Study the drawing (mm; zero at the part's minimum x, y, z) and answer. A direction names the side the tool comes from. Coordinates: 2 decimals unless noted, no trailing zeros. Order: outer loops, then holes, each group sorted by start corner. A loop starts at its lowest first (then second) coordinate and runs counter-clockwise, first axis right, second up. Notation, with made-up numbers: (88, 5.25) -> (101, 5.25) arc R17 ccw to (101, 36.25) -> close; hole circle Ø1 at (45, 71.5). An arc over 180 degrees is marked (long way). One line per question, with ' | ' between items.
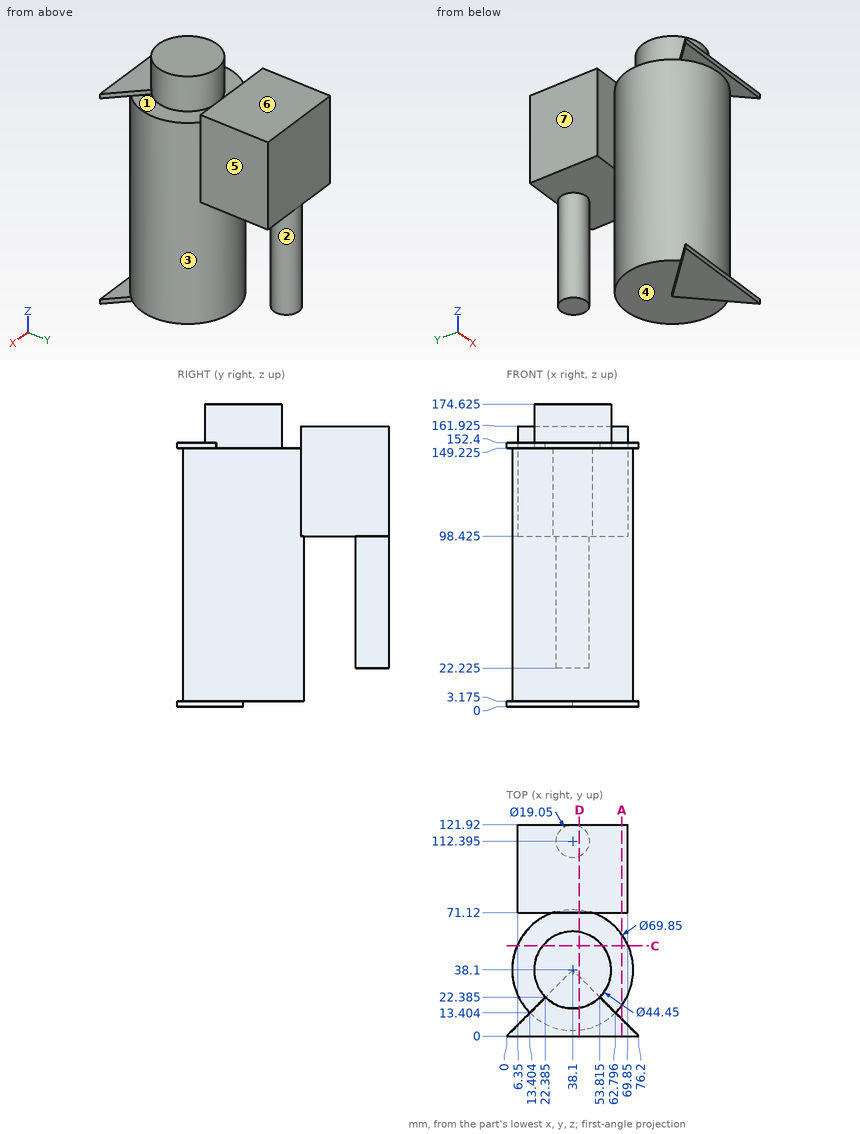
Item 1: Each of these flat-tipped pins is pushed along its axis until it touches: pin 1 Ø1.5 at (y, z) = (30, 156.5) entering from +X (1 decimal); pin 2 Ø10.5 at (x, y) = (52.5, 4.5) entering from -Z; pin 3 Ø1.5 at (y, z) = (55, 22) entering from +X; pin 4 Ø6 at (x, z) = (10.5, 60.5) entering from -Y. Where does it stop, or does it pass through?
Computed values:
pin 1: stops at x = 59.1 | pin 2: stops at z = 0 | pin 3: stops at x = 69.07 | pin 4: stops at y = 13.31
Item 2: For the marked faces 4, 5, 6 and 7, determine the directions among +Z, -Z, +X, -X, +Y, -Y from which every point of the face is accessible in a straight line to the end or side of a thin tool.
Computed values:
face 4: -Z, +Y | face 5: +Z, -Z, +X, +Y | face 6: +Z, +X, -X, +Y | face 7: +Z, -Z, -X, +Y
Item 3: Determine the mould class of the marked faces 1, 2 and 3 for opening direction Z: pulls with the +Z half, pulls with the -Z half, needs draft (parallel to the pull), parting line crosses it, or undercut.
Computed values:
face 1: pulls with the +Z half | face 2: needs draft | face 3: undercut
Item 4: Section D-D, the plane x = 42 is taken. Give the vertices of the cut face in (y, z) (1 decimal), plus the area to 3 significant figures.
Computed values:
outline: (0, 0) -> (34.2, 0) -> (34.2, 3.2) -> (72.8, 3.2) -> (72.8, 98.4) -> (103.7, 98.4) -> (103.7, 22.2) -> (121.1, 22.2) -> (121.1, 98.4) -> (121.9, 98.4) -> (121.9, 161.9) -> (71.1, 161.9) -> (71.1, 149.2) -> (60, 149.2) -> (60, 174.6) -> (16.2, 174.6) -> (16.2, 152.4) -> (0, 152.4) -> (0, 149.2) -> (3.4, 149.2) -> (3.4, 3.2) -> (0, 3.2) -> close | area: 15,900 mm^2
Item 5: Section C-C, the plane y = 52 is taken. Give the vertices of the cut face in (x, z) (1 decimal), plus the area to 3 significant figures.
Computed values:
outline: (6.1, 3.2) -> (70.1, 3.2) -> (70.1, 149.2) -> (55.4, 149.2) -> (55.4, 174.6) -> (20.8, 174.6) -> (20.8, 149.2) -> (6.1, 149.2) -> close | area: 10,200 mm^2
Item 6: Find the intervals of material crossed by L1, parallel to Y at x = 39, z = 66.5; L2, parallel to Z at x = 68, y = 8 (1 decimal); L3, parallel to X at y = 93, z = 123, in increasing order.
Computed values:
L1: y = 3.19 to 73.01, 102.91 to 121.88 | L2: z = 0 to 3.2, 149.2 to 152.4 | L3: x = 6.35 to 69.85
Item 7: Section A-A, the plane x = 66.5 is taken. Give the vertices of the cut face in (y, z) (1 decimal).
Computed values:
outline: (0, 0) -> (9.7, 0) -> (9.7, 3.2) -> (0, 3.2) -> close; (0, 149.2) -> (9.7, 149.2) -> (9.7, 152.4) -> (0, 152.4) -> close; (17.8, 3.2) -> (58.4, 3.2) -> (58.4, 149.2) -> (17.8, 149.2) -> close; (71.1, 98.4) -> (121.9, 98.4) -> (121.9, 161.9) -> (71.1, 161.9) -> close
